Can you work these out from the model? Positions are in its coordinate system, mm. Face numbers are marked on the shaded views. A direction names the side the tool comes from. Coordinates: 2 decimals unless noted, no trailing zeros. Loops run counter-clockwise (first coordinate to the right, second up) from the corner with the lowest first, then second, coordinate; pieces in that order, holes last. Notation, with made-up numbers: (11.25, 37) -> (21.25, 37) arc R20 ccw to (21.25, 52) -> close; hole circle Ø8 at (6, -28). An arc over 180 degrees is marked (long way). Put each result on its own line as item: value. Start each with the question number.
Item 1: Please list where these lines run through material, in increasing order: L1, parallel to X at y = -0.75, z = 4.5; L2, parallel to Z at x = 2, y = -1.5; L3, parallel to Y at x = 1, z = 4.5. Write a range as from..to.
Item 2: Will these pins go through, and if not, where does the flat tip stop? P1, Ø4, axis at y = 1.5, z = -3, coming from the +X side; P2, Ø1.9, axis at x = 2, y = -1.5, coming from the -Z side; P3, Ø0.5, axis at x = 2.5, y = -1.5, coming from the +Z side.
Item 3: If we section it at B-B on x = -0.25: Please give me the cut outline in (y, z), plus the area to 3 significant figures.
Item 4: We'd pull the mould along Y, two halves only. Please class the marked faces 1, 2 and 3: pulls with the +Y half, pulls with the -Y half, needs draft (parallel to the pull), parting line crosses it, or undercut.
Item 5: For the marked faces 4, 5, 6 and 7, which set-ups out of +Z, -Z, +X, -X, +Y, -Y let a thin tool reach every point of the face, with its end or its side?
Item 6: If we section it at A-A on x = 3.75: Please give me the cut outline in (y, z).
```python
from build123d import *

# Parameters (mm, degrees)
F1_DEPTH    = 2
F2_DEPTH    = 5
F3_C1_SIZE  = 0.5
F3_C2_SIZE  = 0.5
F3_C3_SIZE  = 0.5
F3_C4_SIZE  = 0.5
F3_C5_SIZE  = 0.5
F3_C6_SIZE  = 0.5
F3_C7_SIZE  = 0.5
F3_C8_SIZE  = 0.5
F3_C9_SIZE  = 0.5
F3_C10_SIZE = 0.5


with BuildPart() as f1:
    # F0 (on Right) → F1 (new body)
    with BuildSketch(Plane.YZ):
        with BuildLine():
            Line((4.6591372722, 1.30894838), (5.2096475294, 1.30894838))
            Line((5.2096475294, 1.30894838), (5.2096475294, 7.2676605325))
            Line((5.2096475294, 7.2676605325), (-0.7903524706, 9.7676605325))
            Line((-0.7903524706, 9.7676605325), (-1.7747698447, 9.3573516256))
            ThreePointArc((-1.7747698447, 9.3573516256), (-2.2419413153, 6.578748784), (-5.0505708614, 6.3540645439))
            Line((-5.0505708614, 6.3540645439), (-5.5224032781, 5.3671410452))
            Line((-5.5224032781, 5.3671410452), (-5.5224032781, -6.0076899798))
            Line((-5.5224032781, -6.0076899798), (-4.2903524706, -9.2323394675))
            Line((-4.2903524706, -9.2323394675), (5.2096475294, -9.2323394675))
            Line((5.2096475294, -9.2323394675), (5.2096475294, -3.273627315))
            Line((5.2096475294, -3.273627315), (4.6591372722, -3.273627315))
            ThreePointArc((4.6591372722, -3.273627315), (-1.1444544368, -0.9823394675), (4.6591372722, 1.30894838))
        make_face()
        Polygon((-0.058301663, -6.2323394675), (-0.9243270668, -7.7323394675), (-2.6563778744, -7.7323394675), (-3.5224032781, -6.2323394675), (-2.6563778744, -4.7323394675), (-0.9243270668, -4.7323394675), align=None, mode=Mode.SUBTRACT)
        Polygon((-0.2736675582, 5.93383392), (1.1026635838, 6.9853626109), (2.7014797138, 6.3191892234), (2.9239647019, 4.601487145), (1.54763356, 3.5499584541), (-0.0511825701, 4.2161318417), align=None, mode=Mode.SUBTRACT)
        Polygon((-2.6563778744, -7.7323394675), (-0.9243270668, -7.7323394675), (-0.058301663, -6.2323394675), (-0.9243270668, -4.7323394675), (-2.6563778744, -4.7323394675), (-3.5224032781, -6.2323394675), align=None)
        Polygon((2.7014797138, 6.3191892234), (1.1026635838, 6.9853626109), (-0.2736675582, 5.93383392), (-0.0511825701, 4.2161318417), (1.54763356, 3.5499584541), (2.9239647019, 4.601487145), align=None)
    extrude(amount=-F1_DEPTH)

    # F0 (on Right) → F2 (join)
    with BuildSketch(Plane.YZ):
        Polygon((2.7014797138, 6.3191892234), (1.1026635838, 6.9853626109), (-0.2736675582, 5.93383392), (-0.0511825701, 4.2161318417), (1.54763356, 3.5499584541), (2.9239647019, 4.601487145), align=None)
        Polygon((-2.6563778744, -7.7323394675), (-0.9243270668, -7.7323394675), (-0.058301663, -6.2323394675), (-0.9243270668, -4.7323394675), (-2.6563778744, -4.7323394675), (-3.5224032781, -6.2323394675), align=None)
    extrude(amount=F2_DEPTH)

    # F3: chamfer of 0.5 on 12 edges, made by hand

    # F3_c1
    f3_c1_edges = [f1.edges().sort_by_distance(p)[0] for p in [
        (-2, -1.1444544368, -0.9823394675),
    ]]
    chamfer(f3_c1_edges, length=F3_C1_SIZE)

    # F3_c2
    f3_c2_edges = [f1.edges().sort_by_distance(p)[0] for p in [
        (-2, 5.2096475294, 4.352423109),
    ]]
    chamfer(f3_c2_edges, length=F3_C2_SIZE)

    # F3_c3
    f3_c3_edges = [f1.edges().sort_by_distance(p)[0] for p in [
        (-2, 1.9596475294, 8.6218271992),
    ]]
    chamfer(f3_c3_edges, length=F3_C3_SIZE)

    # F3_c4
    f3_c4_edges = [f1.edges().sort_by_distance(p)[0] for p in [
        (-2, -1.6075076826, 9.4270671311),
    ]]
    chamfer(f3_c4_edges, length=F3_C4_SIZE)

    # F3_c5
    f3_c5_edges = [f1.edges().sort_by_distance(p)[0] for p in [
        (-2, -2.43546855, 6.4198809023),
    ]]
    chamfer(f3_c5_edges, length=F3_C5_SIZE)

    # F3_c6
    f3_c6_edges = [f1.edges().sort_by_distance(p)[0] for p in [
        (-2, -5.39514647, 5.633321854),
    ]]
    chamfer(f3_c6_edges, length=F3_C6_SIZE)

    # F3_c7
    f3_c7_edges = [f1.edges().sort_by_distance(p)[0] for p in [
        (-2, -5.5224032781, -0.8998828859),
    ]]
    chamfer(f3_c7_edges, length=F3_C7_SIZE)

    # F3_c8
    f3_c8_edges = [f1.edges().sort_by_distance(p)[0] for p in [
        (-2, -4.6563778744, -8.2743403139),
    ]]
    chamfer(f3_c8_edges, length=F3_C8_SIZE)

    # F3_c9
    f3_c9_edges = [f1.edges().sort_by_distance(p)[0] for p in [
        (-2, 0.7272736227, -9.2323394675),
    ]]
    chamfer(f3_c9_edges, length=F3_C9_SIZE)

    # F3_c10
    f3_c10_edges = [f1.edges().sort_by_distance(p)[0] for p in [
        (-2, 5.2096475294, -6.067102044),
    ]]
    chamfer(f3_c10_edges, length=F3_C10_SIZE)


solid = f1.part
```
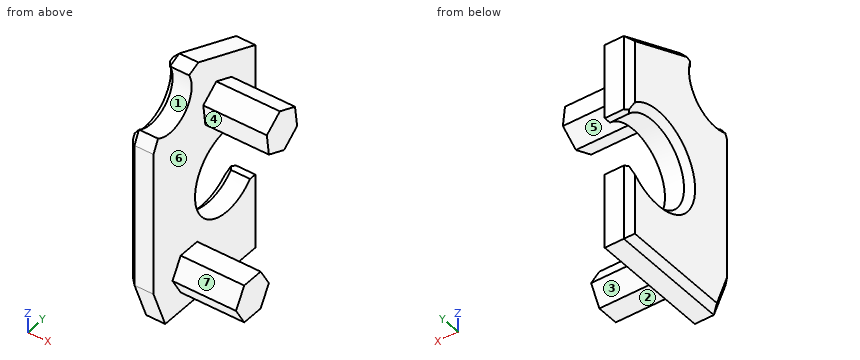
Solutions:
1. L1: -2..0
1. L2: -7.73..-4.73
1. L3: -0.09..2.79
2. P1: x = 0
2. P2: z = -7.73
2. P3: z = -4.73
3. outline: (-5.52, -6.01) -> (-4.29, -9.23) -> (5.21, -9.23) -> (5.21, -3.27) -> (4.66, -3.27) arc R3.35 cw (long way) to (4.66, 1.31) -> (5.21, 1.31) -> (5.21, 7.27) -> (-0.79, 9.77) -> (-1.77, 9.36) arc R2.29 cw to (-5.05, 6.35) -> (-5.52, 5.37) -> close
3. area: 145 mm^2
4. face 1: undercut
4. face 2: needs draft
4. face 3: pulls with the +Y half
5. face 4: +X, -Y
5. face 5: -Z, +X, +Y
5. face 6: +X
5. face 7: +Z, +X, -Y
6. outline: (-3.52, -6.23) -> (-2.66, -7.73) -> (-0.92, -7.73) -> (-0.06, -6.23) -> (-0.92, -4.73) -> (-2.66, -4.73) -> close; (-0.27, 5.93) -> (-0.05, 4.22) -> (1.55, 3.55) -> (2.92, 4.6) -> (2.7, 6.32) -> (1.1, 6.99) -> close
